Model file for the job. Use its own axes, mm. Face numbers are marked on the shaded views. A direction names the side the tool comes from. Give positions to 0.01 mm unless a question says otherwise; leave off trailing zeros. Write each loop counter-clockwise with the first axis right and the second up, starting at its lowest first coordinate (ties: lowest second). Pieces come first, ordered by that corner, then holes. Notation, with made-up numbers: (43.25, 77.5) - (65.25, 77.5) arc R19 cw to (65.25, 101.5) - close; hole circle Ø11 at (41.5, 58.25). An arc over 180 degrees is marked (long way). Use CSV: the item, a comma, the result in double quotes.
from build123d import *
from OCP.BRepFilletAPI import BRepFilletAPI_MakeChamfer

# Parameters (mm, degrees)
SKETCH_1_W          = 45
SKETCH_1_H          = 20
EXTRUDE_1_DEPTH     = 8
CUT_EXTRUDE_1_DEPTH = 2
CUT_EXTRUDE_2_DEPTH = 1
CHAMFER_1_SIZE      = 1
CHAMFER_2_SIZE      = 1
CHAMFER_2_SIZE_2    = 1.732050808
FILLET_1_R          = 1


with BuildPart() as part:
    # 草图1 → 凸台-拉伸1 (new body)
    with BuildSketch(Plane(origin=(0, 0, 0), x_dir=(1, 0, 0), z_dir=(0, 1, 0))):
        with Locations((22.5, 10)):
            Rectangle(SKETCH_1_W, SKETCH_1_H)
        with BuildLine():
            Line((19, 6.7), (8, 6.7))
            ThreePointArc((8, 6.7), (4.7, 10), (8, 13.3))
            Line((8, 13.3), (19, 13.3))
            ThreePointArc((19, 13.3), (22.3, 10), (19, 6.7))
        make_face(mode=Mode.SUBTRACT)
    extrude(amount=EXTRUDE_1_DEPTH)

    # 草图2 → 切除-拉伸1 (cut)
    with BuildSketch(Plane.XZ):
        with BuildLine():
            Line((45, -6.7), (45, -13.3))
            Line((45, -13.3), (8, -13.3))
            ThreePointArc((8, -13.3), (4.7, -10), (8, -6.7))
            Line((8, -6.7), (45, -6.7))
        make_face()
    extrude(amount=-CUT_EXTRUDE_1_DEPTH, mode=Mode.SUBTRACT)

    # 草图3 → 切除-拉伸2 (cut)
    with BuildSketch(Plane.XZ):
        Polygon((0, -6.7), (4.7, -6.7), (4.7, 0), (11.3, 0), (11.3, -20), (4.7, -20), (4.7, -13.3), (0, -13.3), align=None)
    extrude(amount=-CUT_EXTRUDE_2_DEPTH, mode=Mode.SUBTRACT)

    # 倒角1
    chamfer_1_edges = [part.edges().sort_by_distance(p)[0] for p in [
        (0, 0, -16.65),
        (4.7, 0, -16.65),
        (4.7, 0, -3.35),
        (0, 0, -3.35),
    ]]
    chamfer(chamfer_1_edges, length=CHAMFER_1_SIZE - 0.0001)  # a hair under: the kernel refuses the full size

    # 倒角2
    chamfer_2_edges_1 = [part.edges().sort_by_distance(p)[0] for p in [
        (11.3, 0, -16.65),
    ]]
    chamfer_2_side_1 = [part.faces().sort_by_distance(p)[0] for p in [
        (11.3, 0.02, -16.65),
    ]]
    chamfer_2_edges_2 = [part.edges().sort_by_distance(p)[0] for p in [
        (11.3, 0, -3.35),
    ]]
    chamfer_2_side_2 = [part.faces().sort_by_distance(p)[0] for p in [
        (11.3, 0.02, -3.35),
    ]]
    chamfer_2 = BRepFilletAPI_MakeChamfer(part.part.solid().wrapped)
    for e in chamfer_2_edges_1:
        chamfer_2.Add(CHAMFER_2_SIZE - 0.0001, CHAMFER_2_SIZE_2 - 0.0001, e.wrapped, chamfer_2_side_1[0].wrapped)
    for e in chamfer_2_edges_2:
        chamfer_2.Add(CHAMFER_2_SIZE - 0.0001, CHAMFER_2_SIZE_2 - 0.0001, e.wrapped, chamfer_2_side_2[0].wrapped)
    add(Compound.cast(chamfer_2.Shape()), mode=Mode.REPLACE)  # a hair under: the kernel refuses the full size

    # 圆角1
    fillet_1_edges = [part.edges().sort_by_distance(p)[0] for p in [
        (22.5, 8, -20),
        (45, 8, -10),
        (22.5, 8, 0),
        (0, 8, -10),
        (45, 4, 0),
        (45, 4, -20),
        (0, 4.49995, -20),
        (0, 4.49995, 0),
        (45, 0, -16.65),
        (45, 0, -3.35),
    ]]
    fillet(fillet_1_edges, radius=FILLET_1_R)


solid = part.part
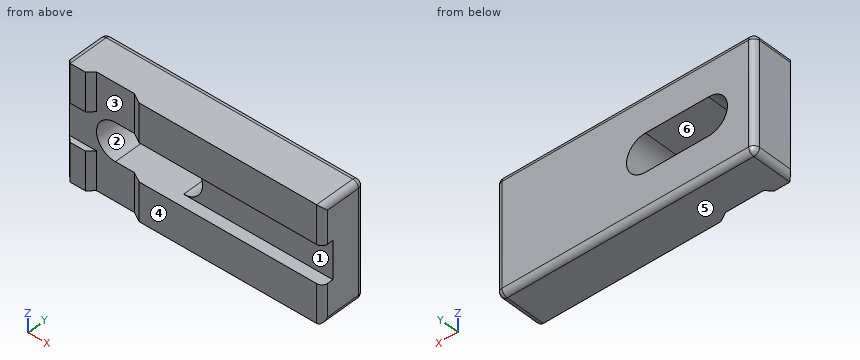
(1) Saw through at C-C, the plane y = 3.25. List the corners of the cut face in (x, z).
Checked values:
outline,"(0, -19) arc R1 ccw to (1, -20) - (44, -20) arc R1 ccw to (45, -19) - (45, -1) arc R1 ccw to (44, 0) - (1, 0) arc R1 ccw to (0, -1) - close; hole (8, -13.3) - (19, -13.3) arc R3.3 ccw to (19, -6.7) - (8, -6.7) arc R3.3 ccw to start"
(2) Pull direction Z, two halves, no side cores. Call the marked faces 4, 5 and 6: released by +Z, released by -Z, zero draft, split by the parting line, or undercut.
Checked values:
face 4,"zero draft"
face 5,"released by -Z"
face 6,"undercut"
(3) Flat gauge pins, fed straight in: P1, Ø12, axis at x = 12, z = -15.5, coming from the -Y side; P2, Ø5.5, axis at x = 35, z = -10, coming from the -Y side. Where does each tip first touch, or does it go through?
Checked values:
P1,"stops at y = 0"
P2,"stops at y = 2"
(4) Saw through at B-B, the plane z = -10. List the corners of the cut face in (x, y), then the cut area to 3 significant figures.
Checked values:
outline,"(0, 1) - (4.7, 1) - (4.7, 8) - (1, 8) arc R1 ccw to (0, 7) - close; (22.3, 2) - (45, 2) - (45, 7) arc R1 ccw to (44, 8) - (22.3, 8) - close"
area,"169 mm^2"
(5) 3-axis set-ups, long thin cutter, end or side, ignore diameter. For the marked faces 1, 2 and 3: which of +Z, -Z, +X, -X, +Y, -Y reach the whole face in a straight line?
Checked values:
face 1,"+X, -Y"
face 2,"+Y, -Y"
face 3,"-Y"
(6) Saw through at A-A, the plane x = 18. List the corners of the cut face in (y, z), then the cut area to 3 significant figures.
Checked values:
outline,"(0, -20) - (7, -20) arc R1 ccw to (8, -19) - (8, -13.3) - (0, -13.3) - close; (0, -6.7) - (8, -6.7) - (8, -1) arc R1 ccw to (7, 0) - (0, 0) - close"
area,"107 mm^2"
(7) Wall check: probe 1 along Y at (x, z) = (25, -8.25); probe 2 along X at (y, z) = (4.5, -7.75); probe 3 along Z at (x, y) = (12, 1). Give the ranges that are in metal, low to high. Write a range as [from, to].
Checked values:
probe 1,"y = [2, 8]"
probe 2,"x = [0, 5.59], [21.41, 45]"
probe 3,"z = [-20, -13.3], [-6.7, 0]"
